```python
from build123d import *

# Parameters (mm, degrees)
SKETCH1_R           = 5
SKETCH1_R_2         = 4
BOSS_EXTRUDE1_DEPTH = 5
FILLET3_R           = 5


with BuildPart() as part:
    # Sketch1 → Boss-Extrude1 (new body)
    with BuildSketch(Plane.XY):
        with BuildLine():
            Line((-10, 10), (10, 10))
            Line((10, 10), (10, -10))
            Line((10, -10), (-10, -10))
            ThreePointArc((-10, -10), (-80.710678119, 19.289321881), (-110, 90))
            Line((-110, 90), (-110, 160))
            Line((-110, 160), (-90, 160))
            Line((-90, 160), (-90, 90))
            ThreePointArc((-90, 90), (-89.975789808, 88.031994787), (-89.903173887, 86.065180718))
            Line((-89.903173887, 86.065180718), (-71.639655664, 89.285531744))
            Line((-71.639655664, 89.285531744), (-66.94119256, 90.99563246))
            Line((-66.94119256, 90.99563246), (-65.231091843, 86.297169356))
            Line((-65.231091843, 86.297169356), (-69.929554947, 84.58706864))
            Line((-69.929554947, 84.58706864), (-68.732484445, 81.298144467))
            Line((-68.732484445, 81.298144467), (-71.551562308, 80.272084037))
            Line((-71.551562308, 80.272084037), (-71.927784465, 81.30574592))
            Line((-71.927784465, 81.30574592), (-74.089077493, 80.51909959))
            Line((-74.089077493, 80.51909959), (-73.712855336, 79.485437707))
            Line((-73.712855336, 79.485437707), (-78.129410653, 77.877943034))
            Line((-78.129410653, 77.877943034), (-77.103350223, 75.058865171))
            Line((-77.103350223, 75.058865171), (-72.686794906, 76.666359845))
            Line((-72.686794906, 76.666359845), (-72.310572748, 75.632697962))
            Line((-72.310572748, 75.632697962), (-70.14927972, 76.419344292))
            Line((-70.14927972, 76.419344292), (-70.525501878, 77.453006175))
            Line((-70.525501878, 77.453006175), (-67.706424015, 78.479066605))
            Line((-67.706424015, 78.479066605), (-66.509353514, 75.190142432))
            Line((-66.509353514, 75.190142432), (-61.81089041, 76.900243149))
            Line((-61.81089041, 76.900243149), (-60.100789693, 72.201780045))
            Line((-60.100789693, 72.201780045), (-64.799252797, 70.491679328))
            Line((-64.799252797, 70.491679328), (-64.693728557, 70.201753861))
            Line((-64.693728557, 70.201753861), (-86.430210334, 66.369025658))
            ThreePointArc((-86.430210334, 66.369025658), (-57.484324006, 25.616469702), (-10, 10))
        make_face()
        Circle(SKETCH1_R, mode=Mode.SUBTRACT)
        with Locations((-100, 150)):
            Circle(SKETCH1_R_2, mode=Mode.SUBTRACT)
    extrude(amount=BOSS_EXTRUDE1_DEPTH)

    # Fillet3
    # the kernel refuses this fillet: 5 mm, written as the material it adds along each edge
    with BuildSketch(Plane(origin=(-86.430210334, 66.369025658, 0), x_dir=(0.9848077530122086, 0.17364817766692744, 0), z_dir=(0, 0, 1))) as fillet3_piece_1:
        with BuildLine():
            CenterArc((5.887847048, -5), FILLET3_R, 90, 101.536959033)
            ThreePointArc((0.988867563, -6), (0.437404346, -3.009399093), (0, 0))
            Line((0, 0), (5.887847048, 0))
        make_face()
    extrude(amount=5)
    with BuildSketch(Plane(origin=(-89.903173887, 86.065180718, 0), x_dir=(-0.01629387917599103, 0.9998672459388787, 0), z_dir=(0, 0, 1))) as fillet3_piece_2:
        with BuildLine():
            CenterArc((5.8610144, -4.99933623), FILLET3_R, 89.066388177, 100)
            Line((0.923482309, -5.787230163), (0.4297291, -5.866019556))
            Line((0.4297291, -5.866019556), (-0.493753209, -0.078789393))
            Line((-0.493753209, -0.078789393), (-0.016452277, 0.499729249))
            ThreePointArc((-0.016452277, 0.499729249), (3.944021531, 0.532633412), (5.950630735, 0.499933623))
            Line((5.950630735, 0.499933623), (5.942483796, 0))
        make_face()
    extrude(amount=5)
    # the kernel refuses this fillet: 5 mm, written as the material it takes off along each edge
    with BuildSketch(Plane(origin=(10, -10, -12.5), x_dir=(0, 1, 0), z_dir=(0, 0, 1)), Plane(origin=(10, 10, -12.5), x_dir=(-1, 0, 0), z_dir=(0, 0, 1))) as fillet3_2_piece_1:
        with BuildLine():
            CenterArc((FILLET3_R, FILLET3_R), FILLET3_R, 180, 90)
            Line((0, FILLET3_R), (0, 0))
            Line((0, 0), (FILLET3_R, 0))
        make_face()
    extrude(amount=30, mode=Mode.SUBTRACT)
    with BuildSketch(Plane(origin=(-90, 160, -12.5), x_dir=(0, -1, 0), z_dir=(0, 0, 1)), Plane(origin=(-110, 160, -12.5), x_dir=(1, 0, 0), z_dir=(0, 0, 1))) as fillet3_2_piece_2:
        with BuildLine():
            CenterArc((FILLET3_R, -FILLET3_R), FILLET3_R, 90, 90)
            Line((0, -FILLET3_R), (0, 0))
            Line((0, 0), (FILLET3_R, 0))
        make_face()
    extrude(amount=30, mode=Mode.SUBTRACT)
    with BuildSketch(Plane(origin=(-64.693728557, 70.201753861, -4.425012024), x_dir=(-0.9848077530122087, -0.17364817766692653, 0), z_dir=(0, 0, 1))) as fillet3_2_piece_3:
        with BuildLine():
            CenterArc((1.77000481, -5), FILLET3_R, 90, 20.077186637)
            Line((0.053576061, -0.30384494), (0, 0))
            Line((0, 0), (1.77000481, 0))
        make_face()
    extrude(amount=13.850024049, mode=Mode.SUBTRACT)


solid = part.part
```
Could you check a few things on this model? Use its own coordinates, in mm. A direction names the side the tool comes from. Coordinates: 2 decimals unless noted, no trailing zeros. Write each loop counter-clockwise with the first axis right and the second up, starting at its lowest first coordinate (ties: lowest second). Pieces come first, ordered by that corner, then holes. Notation, with made-up numbers: (26, 14) -> (57, 14) arc R19 cw to (57, 34) -> close; hole circle Ø4 at (45, 68). An arc over 180 degrees is marked (long way). Write item = value, one per line. Start each with the question number.
(1) We'd pull the mould along Y, two halves only. Please class faces 1 (the face through (-69.34, 82.97, 2.46)), 2 (the face through (-77, 69, 0)), 3 (the face through (-60.968, 74.584, 2.465)), 4 (the face through (-74.93, 75.85, 2.46)): released by +Y, released by -Y, zero draft, split by the parting line, or undercut.
(2) I want a section at A-A (y = 150). Please give me the cut outline in (x, z).
(3) Which directions (+Z, -Z, +X, -X, +Y, -Y) give clear straight access to the entire face, cutting with the end or side of a thin tool? Please do faces 5 (the face through (-67.116, 76.858, 2.465)), 6 (the face through (-77.97, 88.17, 2.46)), 7 (the face through (-62.417, 71.359, 2.465)).
(4) I want a section at B-B (x = 0). Please give me the cut outline in (y, z).
(5) I need wall thicknesses on line 1 (Y direction, x = 0, z = 1.9); line 2 (Y direction, x = -71, z = 2); line 3 (X direction, y = 93.5, z = 3.3). Which ranges of each line are inside material? Lowest first, please. Write a range as [from, to].
(6) I want a section at D-D (y = 118). Please give me the cut outline in (x, z).
(7) Will these pins go through, and if not, where does the flat tip stop? pin 1 (2.5 mm diameter, centred on y = 111.5, z = 2, fed in from +X); pin 2 (1.5 mm diameter, centred on y = 32, z = 4, fed in from -X); pin 3 (3 mm diameter, centred on x = -88, z = 4.5, fed in from -Y); pin 4 (11.5 mm diameter, centred on x = 0, y = 0, fed in from +Z).
(8) I want a section at C-C (z = 2.9). Give the number of separate pieces and of enclosed holes in the cut face, plus the area to 3 significant figures.
Result set:
q1.face_1 = undercut
q1.face_2 = zero draft
q1.face_3 = released by +Y
q1.face_4 = undercut
q2.outline = (-110, 0) -> (-104, 0) -> (-104, 5) -> (-110, 5) -> close; (-96, 0) -> (-90, 0) -> (-90, 5) -> (-96, 5) -> close
q3.face_5 = +Z, -Z
q3.face_6 = +Z, -Z, +Y
q3.face_7 = +Z, -Z, +X
q4.outline = (-10, 0) -> (-5, 0) -> (-5, 5) -> (-10, 5) -> close; (5, 0) -> (10, 0) -> (10, 5) -> (5, 5) -> close
q5.line_1 = [-10, -5], [5, 10]
q5.line_2 = [10.76, 38.24], [69.09, 76.11], [80.47, 89.52]
q5.line_3 = [-110, -90]
q6.outline = (-110, 0) -> (-90, 0) -> (-90, 5) -> (-110, 5) -> close
q7.pin_1 = -90
q7.pin_2 = -91.99
q7.pin_3 = 25.6
q7.pin_4 = 5
q8.separate_pieces = 1
q8.enclosed_holes = 2
q8.area = 4,920 mm2
